The figure shows three views and two pictorial views of one solid part (mm, origin at its lowest corner). Answer the questions. Coordinates: 2 decimals unless noted, no trailing zeros. Write each loop counter-clockwise with the first axis right and the second up, starting at its lowest first coordinate (ties: lowest second). Pieces come first, ordered by that corner, then holes. Notation, with made-up numbers: M 56.5,48 L 109.5,48 A34 ccw 109.5,85 Z; hole C 26,-3.5 d11. An arc over 180 degrees is marked long. Use CSV: the item, a comma, the result in double quotes.
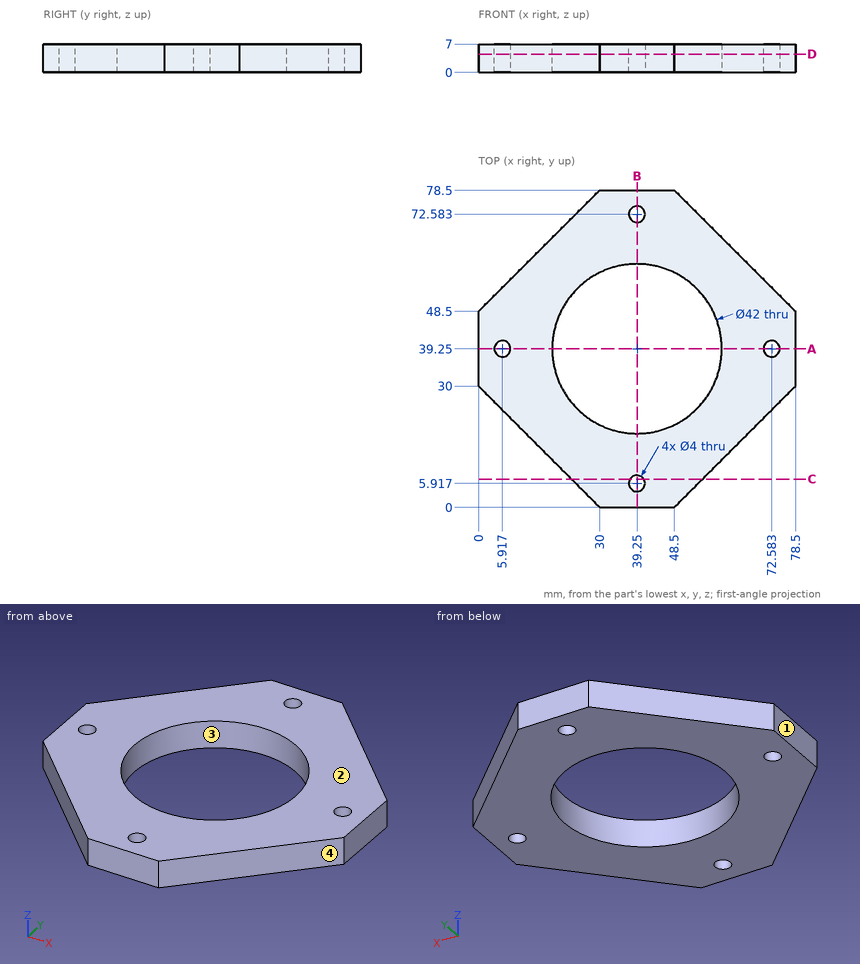
Item 1: The part is cut by section C-C (y = 7). Write down the section's boundary in (x, z).
Answer:
outline,"M 23,0 L 37.57,0 L 37.57,7 L 23,7 Z; M 40.93,0 L 55.5,0 L 55.5,7 L 40.93,7 Z"
Item 2: Consider probe 1 along Y at (x, z) = (39.25, 1.5); probe 2 along X at (y, z) = (53, 6); probe 3 along Y at (x, z) = (41.5, 0.5). Determine where each line is inside the solid, lowest interval first.
Answer:
probe 1,"y = 0 to 3.92, 7.92 to 18.25, 60.25 to 70.58, 74.58 to 78.5"
probe 2,"x = 4.5 to 23.38, 55.12 to 74"
probe 3,"y = 0 to 18.37, 60.13 to 78.5"
Item 3: The part is cut by section A-A (y = 39.25). Write down the section's boundary in (x, z).
Answer:
outline,"M 0,0 L 3.92,0 L 3.92,7 L 0,7 Z; M 7.92,0 L 18.25,0 L 18.25,7 L 7.92,7 Z; M 60.25,0 L 70.58,0 L 70.58,7 L 60.25,7 Z; M 74.58,0 L 78.5,0 L 78.5,7 L 74.58,7 Z"
Item 4: Given pin 1 (3.5 mm diameter, centred on x = 5.92, y = 39.25, fed in from +Z); pin 2 (3 mm diameter, centred on x = 54.5, z = 1, fed in from +Y); pin 3 (2 mm diameter, centred on y = 54, z = 6.5, fed in from -X), each flat-ended and moving along its own axis, determine where each tip first touches the part or whether it passes through.
Answer:
pin 1,"passes through"
pin 2,"stops at y = 74"
pin 3,"stops at x = 4.5"
Item 5: The part is cut by section D-D (z = 4.5). Write down the section's boundary in (x, y).
Answer:
outline,"M 0,30 L 30,0 L 48.5,0 L 78.5,30 L 78.5,48.5 L 48.5,78.5 L 30,78.5 L 0,48.5 Z; hole C 5.92,39.25 d4; hole C 39.25,39.25 d42; hole C 39.25,5.92 d4; hole C 39.25,72.58 d4; hole C 72.58,39.25 d4"
Item 6: For a pull along X with two mould halves and no side action, classify the marked faces 1, 2, 3 and 4 as released by +X, released by -X, zero draft, split by the parting line, or undercut.
Answer:
face 1,"released by -X"
face 2,"zero draft"
face 3,"undercut"
face 4,"released by +X"
